Geometry: see drawing. Coordinates: mm, zero at the bounding-box minimum. Round coordinates to 2 decimals unless told otherwise and drop trailing zeros. Write each loop counter-clockwise with the first axis right and the second up, starting at its lowest first coordinate (ties: lowest second). Pieces come first, ordered by that corner, then holes. Notation, with made-up numbers: (12, 43.25) -> (38, 43.25) arc R20 cw to (38, 82.25) -> close; hole circle Ø7 at (-5.75, 34). An arc over 180 degrees is marked (long way). Use CSV: the item, a comma, the result in double quotes.
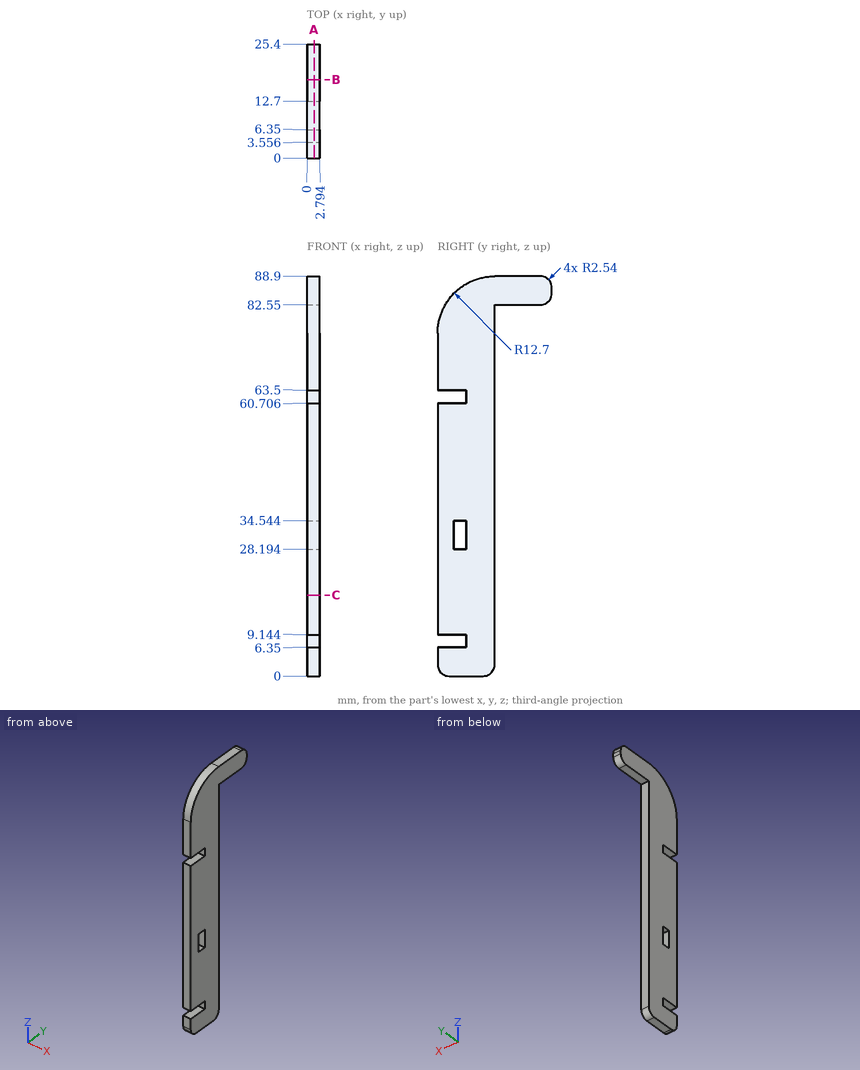
Item 1: Line query: line 1 (Z direction, x = 1.25, y = 23); line 2 (Y direction, x = 1.75, z = 43); line 3 (Z direction, x = 0.7, y = 10.75). Output: solid intervals per line, ascending.
Worked answers:
line 1,"z = 82.55 to 88.9"
line 2,"y = 0 to 12.7"
line 3,"z = 0.07 to 88.75"
Item 2: First-contact query: pin 1 Ø1 at (x, z) = (0.5, 63.5) entering from +Y; pin 2 Ø1.4 at (x, z) = (1, 8) entering from -Y; pin 3 Ø1.5 at (x, y) = (0.5, 11.5) entering from -Z. Flat tips, straight axial feed; report the tip coordinate or a pass-through.
Worked answers:
pin 1,"stops at y = 12.7"
pin 2,"stops at y = 6.35"
pin 3,"stops at z = 0.07"
Item 3: Section query C-C on z = 18. Return the cut outline in (x, y), plus the area to 3 significant figures.
Worked answers:
outline,"(0, 0) -> (2.79, 0) -> (2.79, 12.7) -> (0, 12.7) -> close"
area,"35.5 mm²"
Item 4: Section query A-A on x = 1.55. Return the cut outline in (y, z).
Worked answers:
outline,"(0, 2.54) arc R2.54 ccw to (2.54, 0) -> (10.16, 0) arc R2.54 ccw to (12.7, 2.54) -> (12.7, 82.55) -> (22.86, 82.55) arc R2.54 ccw to (25.4, 85.09) -> (25.4, 86.36) arc R2.54 ccw to (22.86, 88.9) -> (12.7, 88.9) arc R12.7 ccw to (0, 76.2) -> (0, 63.5) -> (6.35, 63.5) -> (6.35, 60.71) -> (0, 60.71) -> (0, 9.14) -> (6.35, 9.14) -> (6.35, 6.35) -> (0, 6.35) -> close; hole (3.56, 28.19) -> (6.35, 28.19) -> (6.35, 34.54) -> (3.56, 34.54) -> close"
Item 5: Section query B-B on y = 17.5. Return the cut outline in (x, z), plus the area to 3 significant figures.
Worked answers:
outline,"(0, 82.55) -> (2.79, 82.55) -> (2.79, 88.9) -> (0, 88.9) -> close"
area,"17.7 mm²"
